Verification items for the finished model (mm, model axes). Face numbers are marked on the shaded views. Coordinates: 2 decimals unless noted, no trailing zeros. Order: outer loops, then holes, each group sorted by start corner. A loop starts at its lowest first (then second) coordinate and runs counter-clockwise, first axis right, second up. Notation, with made-up numbers: M 82.5,-17 L 122.5,-17 A26 cw 122.5,3 Z; hole C 56.25,14 d8. An arc over 180 degrees is marked long. Return JSON: item names as keys, results as strings. Group by question number.
1. Mould release check, pull along Y, two halves, no side actions. Record for the marked faces 1, 2 and 3: +Y half, -Y half, draft (parallel to the pull), parting line (faces both ways), or undercut.
2. Section check B-B, the plane y = 25. Record the cut outline in (x, z).
3. Section check C-C, the plane z = 8.5. Give the number of separate pieces and of enclosed holes in the cut face, plus the area to 3 significant figures.
4. Section check A-A, the plane x = 20. Record the cut outline in (y, z), plus the area to 3 significant figures.
5. Gauge pin test, flat ends, axial feed: pin 1 (12 mm diameter, centred on x = -20, y = 40, fed in from +Z); pin 2 (6.5 mm diameter, centred on x = 0, y = 25, fed in from +Z). Record the tip position at first contact, or that the pin passes through.
6. Section check D-D, the plane y = 0. Record the cut outline in (x, z).
7. Material ranges on line 1 along Y through (x, z) = (-20, 5.25); line 2 along X through (y, z) = (5.5, 2.25); line 3 along Y through (x, z) = (-16, 3.5), recorded low to high.
```python
from build123d import *

# Parameters (mm, degrees)
SKETCH_1_R          = 7.5
SKETCH_1_R_2        = 2.25
EXTRUDE_1_DEPTH     = 10
SKETCH_2_R          = 4
CUT_EXTRUDE_1_DEPTH = 4.4


with BuildPart() as part:
    # 草图1 → 凸台-拉伸1 (new body)
    with BuildSketch(Plane.XY):
        with BuildLine():
            Line((-25, -60), (25, -60))
            ThreePointArc((25, -60), (32.071067812, -57.071067812), (35, -50))
            Line((35, -50), (35, 50))
            ThreePointArc((35, 50), (32.071067812, 57.071067812), (25, 60))
            Line((25, 60), (-25, 60))
            ThreePointArc((-25, 60), (-32.071067812, 57.071067812), (-35, 50))
            Line((-35, 50), (-35, -50))
            ThreePointArc((-35, -50), (-32.071067812, -57.071067812), (-25, -60))
        make_face()
        with Locations((20, 40)):
            Circle(SKETCH_1_R, mode=Mode.SUBTRACT)
        with Locations((20, 0)):
            Circle(SKETCH_1_R, mode=Mode.SUBTRACT)
        with Locations(Location((20, -40, 0), (0, 0, 180))):
            Circle(SKETCH_1_R, mode=Mode.SUBTRACT)
        with Locations((-20, -40)):
            Circle(SKETCH_1_R, mode=Mode.SUBTRACT)
        with Locations(Location((-20, 0, 0), (0, 0, 180))):
            Circle(SKETCH_1_R, mode=Mode.SUBTRACT)
        with Locations(Location((-20, 40, 0), (0, 0, 180))):
            Circle(SKETCH_1_R, mode=Mode.SUBTRACT)
        with Locations((0, 25)):
            Circle(SKETCH_1_R_2, mode=Mode.SUBTRACT)
        with Locations(Location((0, -25, 0), (0, 0, 180))):
            Circle(SKETCH_1_R_2, mode=Mode.SUBTRACT)
    extrude(amount=EXTRUDE_1_DEPTH)

    # 草图2 → 切除-拉伸1 (cut)
    with BuildSketch(Plane.XY.offset(10)):
        with Locations((0, 25)):
            Circle(SKETCH_2_R)
        with Locations((0, -25)):
            Circle(SKETCH_2_R)
    extrude(amount=-CUT_EXTRUDE_1_DEPTH, mode=Mode.SUBTRACT)


solid = part.part
```
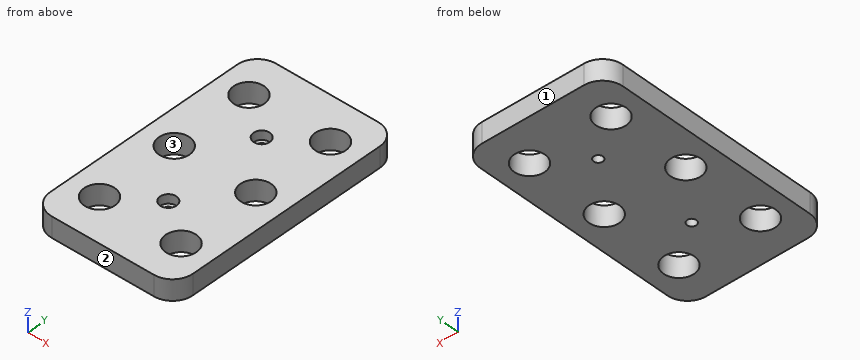
Answers follow:
{
 "1": {"face 1": "+Y half", "face 2": "-Y half", "face 3": "undercut"},
 "2": {"outline": "M -35,0 L -2.25,0 L -2.25,5.6 L -4,5.6 L -4,10 L -35,10 Z; M 2.25,0 L 35,0 L 35,10 L 4,10 L 4,5.6 L 2.25,5.6 Z"},
 "3": {"separate pieces": "1", "enclosed holes": "8", "area": "7,150 mm^2"},
 "4": {"outline": "M -60,0 L -47.5,0 L -47.5,10 L -60,10 Z; M -32.5,0 L -7.5,0 L -7.5,10 L -32.5,10 Z; M 7.5,0 L 32.5,0 L 32.5,10 L 7.5,10 Z; M 47.5,0 L 60,0 L 60,10 L 47.5,10 Z", "area": "750 mm^2"},
 "5": {"pin 1": "through", "pin 2": "z = 5.6"},
 "6": {"outline": "M -35,0 L -27.5,0 L -27.5,10 L -35,10 Z; M -12.5,0 L 12.5,0 L 12.5,10 L -12.5,10 Z; M 27.5,0 L 35,0 L 35,10 L 27.5,10 Z"},
 "7": {"line 1": "-60 to -47.5, -32.5 to -7.5, 7.5 to 32.5, 47.5 to 60", "line 2": "-35 to -25.1, -14.9 to 14.9, 25.1 to 35", "line 3": "-60 to -46.34, -33.66 to -6.34, 6.34 to 33.66, 46.34 to 60"}
}
